Could you check a few things on this model? Use its own coordinates, in mm. A direction names the side the tool comes from. Coordinates: 2 decimals unless noted, no trailing zeros. Order: outer loops, then holes, each group sorted by start corner. A loop starts at its lowest first (then second) coordinate and runs counter-clockwise, first axis right, second up.
```python
from build123d import *

# Parameters (mm, degrees)
SKETCH1_W               = 37.8
SKETCH1_H               = 20.85
BOSS_EXTRUDE1_DEPTH     = 8.5
SKETCH2_W               = 5
SKETCH2_H               = 17.95
BOSS_EXTRUDE2_DEPTH     = 8.5
SKETCH3_W               = 23.2
SKETCH3_H               = 13
CUT_EXTRUDE1_DEPTH      = 18.85
SKETCH4_W               = 1.4
SKETCH4_H               = 13
CUT_EXTRUDE3_DEPTH      = 5.8
CUT_EXTRUDE4_DEPTH      = 33.550729639
CUT_EXTRUDE4_DEPTH_BACK = 33.550729639
SKETCH5_W               = 9.7
SKETCH5_H               = 4
BOSS_EXTRUDE3_DEPTH     = 8.5
SKETCH7_W               = 5.3
SKETCH7_H               = 13
CUT_EXTRUDE5_DEPTH      = 9.85
SKETCH8_R               = 3
BOSS_EXTRUDE4_DEPTH     = 3
SKETCH9_R               = 1.25
CUT_EXTRUDE6_DEPTH      = 4.3
SKETCH10_R              = 1.25
CUT_EXTRUDE7_DEPTH      = 4.3
SKETCH11_R              = 1.5
BOSS_EXTRUDE5_DEPTH     = 2.8


with BuildPart() as part:
    # Sketch1 → Boss-Extrude1 (new, symmetric)
    with BuildSketch(Plane.XY):
        with Locations((-2.4, -5.275)):
            Rectangle(SKETCH1_W, SKETCH1_H)
    extrude(amount=BOSS_EXTRUDE1_DEPTH, both=True)

    # Sketch2 → Boss-Extrude2 (add, symmetric)
    with BuildSketch(Plane.XY):
        with Locations((-18.8, 14.125)):
            Rectangle(SKETCH2_W, SKETCH2_H)
    extrude(amount=BOSS_EXTRUDE2_DEPTH, both=True)

    # Sketch3 → Cut-Extrude1 (cut)
    with BuildSketch(Plane(origin=(0, 5.15, 0), x_dir=(1, 0, 0), z_dir=(0, 1, 0))):
        Rectangle(SKETCH3_W, SKETCH3_H)
    extrude(amount=-CUT_EXTRUDE1_DEPTH, mode=Mode.SUBTRACT)

    # Sketch4 → Cut-Extrude3 (cut)
    with BuildSketch(Plane(origin=(0, -13.7, 0), x_dir=(1, 0, 0), z_dir=(0, 1, 0))):
        with Locations((12.3, 0)):
            Rectangle(SKETCH4_W, SKETCH4_H)
    extrude(amount=CUT_EXTRUDE3_DEPTH, mode=Mode.SUBTRACT)

    # Sketch5 → Cut-Extrude4 (cut, two sides: drawn at the far end of the back side and taken through both)
    with BuildSketch(Plane.XY.offset(-CUT_EXTRUDE4_DEPTH_BACK)):
        with Locations((-16.45, -11.7)):
            Rectangle(SKETCH5_W, SKETCH5_H)
    extrude(amount=CUT_EXTRUDE4_DEPTH + CUT_EXTRUDE4_DEPTH_BACK, mode=Mode.SUBTRACT)

    # Sketch6 → Boss-Extrude3 (add, symmetric)
    with BuildSketch(Plane.XY):
        Polygon((-16.3, 5.15), (-11, 5.15), (-16.3, 15), align=None)
    extrude(amount=BOSS_EXTRUDE3_DEPTH, both=True)

    # Sketch7 → Cut-Extrude5 (cut)
    with BuildSketch(Plane(origin=(0, 15, 0), x_dir=(1, 0, 0), z_dir=(0, 1, 0))):
        with Locations((-13.65, 0)):
            Rectangle(SKETCH7_W, SKETCH7_H)
    extrude(amount=-CUT_EXTRUDE5_DEPTH, mode=Mode.SUBTRACT)

    # Sketch8 → Boss-Extrude4 (add)
    with BuildSketch(Plane(origin=(0, -18.7, 0), x_dir=(1, 0, 0), z_dir=(0, 1, 0))):
        with Locations(Location((5.5, 0, 0), (0, 0, 270))):
            Circle(SKETCH8_R)
    extrude(amount=BOSS_EXTRUDE4_DEPTH)

    # Sketch9 → Cut-Extrude6 (cut)
    with BuildSketch(Plane(origin=(0, 23.1, 0), x_dir=(1, 0, 0), z_dir=(0, 1, 0))):
        with Locations(Location((-18.8, -4.5, 0), (0, 0, 270))):
            Circle(SKETCH9_R)
    extrude(amount=-CUT_EXTRUDE6_DEPTH, mode=Mode.SUBTRACT)

    # Sketch10 → Cut-Extrude7 (cut)
    with BuildSketch(Plane(origin=(0, 23.1, 0), x_dir=(1, 0, 0), z_dir=(0, 1, 0))):
        with Locations(Location((-18.8, 4.5, 0), (0, 0, 270))):
            Circle(SKETCH10_R)
    extrude(amount=-CUT_EXTRUDE7_DEPTH, mode=Mode.SUBTRACT)

    # Sketch11 → Boss-Extrude5 (add)
    with BuildSketch(Plane(origin=(-24.1, 0, 0), x_dir=(0, 0, -1), z_dir=(1, 0, 0))):
        with Locations((-4, -4)):
            Circle(SKETCH11_R)
        with Locations((4, -4)):
            Circle(SKETCH11_R)
        with Locations((-4, 4)):
            Circle(SKETCH11_R)
        with Locations((4, 4)):
            Circle(SKETCH11_R)
    extrude(amount=BOSS_EXTRUDE5_DEPTH)


solid = part.part
```
Item 1: Which directions (+Z, -Z, +X, -X, +Y, -Y) give clear straight access to the entire face, cutting with the end or side of a thin tool? Please do faces 1 (the face through (12, 5.15, 0)), 2 (the face through (-17, -9.7, 0)), 3 (the face through (-22.72, 4.45, 2.57)).
Item 2: Thinking about a two-plate mould opening in X: for faces 4 (the face through (-17.56, 20.98, -4.66)), 5 (the face through (-3, -15.7, 0)), 6 (the face through (2.57, -17.22, -0.65)), 7 (the face through (-24.1, -4, -4)), which applies, +X half, -X half, draft (parallel to the pull), parting line (faces both ways), or undercut?
Item 3: I need wall thicknesses on line 1 (X direction, y = 22.25, z = -4.5); line 2 (Z direction, x = 1, y = -4.5); line 3 (Y direction, x = -18.5, z = -0.5). Which ranges of each line are inside material? Lowest first, please.
Item 4: Suppose I cut it at D-D (x = -4). List the corners of the cut face in (y, z) for me.
Item 5: Suppose I cut it at B-B (y = 4). List the corners of the cut face in (x, z) for me.
Item 6: Suppose I cut it at C-C (x = -18.8). List the corners of the cut face in (y, z) for me, and give its area (3 significant figures).
Item 7: Suppose I cut it at A-A (z = 0). List the corners of the cut face in (x, y) for me, and give its area (3 significant figures).
Item 8: For pin 1 Ø6 at (x, z) = (-9, 0.5) entering from -Y; pin 2 Ø1.5 at (x, z) = (-18.8, 4.5) entering from +Y; pin 3 Ø2 at (y, z) = (-12, 8) entering from -X, each with a flat end and sliding along its axis, tell me the tip position at first contact or that it passes through.
Geometry results:
1. face 1: +Z, -Z, +X, +Y
1. face 2: +Z, -Z, -X
1. face 3: -X
2. face 4: undercut
2. face 5: draft
2. face 6: parting line
2. face 7: -X half
3. line 1: x = -21.3 to -20.05, -17.55 to -16.3
3. line 2: z = -8.5 to -6.5, 6.5 to 8.5
3. line 3: y = -15.7 to -13.7, -9.7 to 23.1
4. outline: (-15.7, -8.5) - (5.15, -8.5) - (5.15, -6.5) - (-13.7, -6.5) - (-13.7, 6.5) - (5.15, 6.5) - (5.15, 8.5) - (-15.7, 8.5) - close
5. outline: (-24.1, -5.5) - (-21.3, -5.5) - (-21.3, -8.5) - (16.5, -8.5) - (16.5, 8.5) - (-21.3, 8.5) - (-21.3, 5.5) - (-24.1, 5.5) - (-24.1, 2.5) - (-21.3, 2.5) - (-21.3, -2.5) - (-24.1, -2.5) - close; hole (-11.6, -6.5) - (11.6, -6.5) - (11.6, 6.5) - (-11.6, 6.5) - close
6. outline: (-15.7, -8.5) - (-13.7, -8.5) - (-13.7, 8.5) - (-15.7, 8.5) - close; (-9.7, -8.5) - (23.1, -8.5) - (23.1, -5.75) - (18.8, -5.75) - (18.8, -3.25) - (23.1, -3.25) - (23.1, 3.25) - (18.8, 3.25) - (18.8, 5.75) - (23.1, 5.75) - (23.1, 8.5) - (-9.7, 8.5) - close
6. area: 570 mm2
7. outline: (-21.3, -15.7) - (2.5, -15.7) - (2.5, -18.7) - (8.5, -18.7) - (8.5, -15.7) - (16.5, -15.7) - (16.5, 5.15) - (11.6, 5.15) - (11.6, -7.9) - (13, -7.9) - (13, -13.7) - (-21.3, -13.7) - close; (-21.3, -9.7) - (-11.6, -9.7) - (-11.6, 5.15) - (-16.3, 5.15) - (-16.3, 23.1) - (-21.3, 23.1) - close
7. area: 412 mm2
8. pin 1: stops at y = -15.7
8. pin 2: stops at y = 18.8
8. pin 3: stops at x = -11.6
